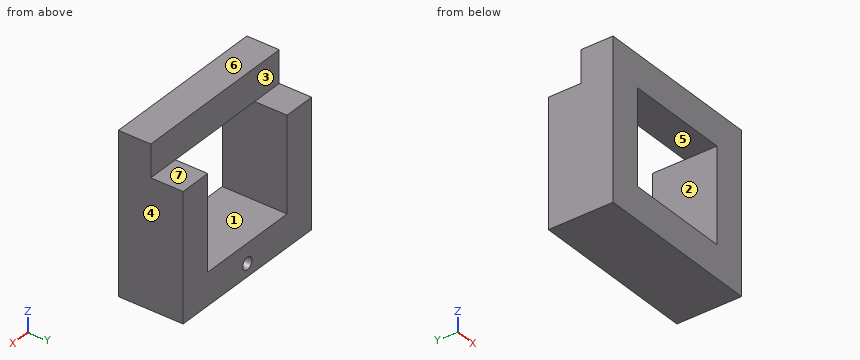
Autodesk Inventor part; units mm, degrees
ref_plane "YZ Plane" through (0, 0, 0) normal (1, 0, 0) x (0, 1, 0)
ref_plane "XZ Plane" through (0, 0, 0) normal (0, 1, 0) x (-1, 0, 0)
ref_plane "XY Plane" through (0, 0, 0) normal (0, 0, 1) x (1, 0, 0)
sketch "Sketch1" plane through (0, 0, 0) normal (0, 1, 0) x (-1, 0, 0)
  line L0 (8.1915, 7.4295) -> (-8.1915, 7.4295)
  line L1 (-8.1915, 7.4295) -> (-8.1915, -7.4295)
  line L2 (-8.1915, -7.4295) -> (8.1915, -7.4295)
  line L3 (8.1915, -7.4295) -> (8.1915, 7.4295)
  line L4 (13.2715, -12.5095) -> (-13.2715, -12.5095)
  line L5 (-13.2715, -12.5095) -> (-13.2715, 12.5095)
  line L6 (-13.2715, 12.5095) -> (13.2715, 12.5095)
  line L7 (13.2715, 12.5095) -> (13.2715, -12.5095)
  point P0 (0, 0)
  point P1 (0, -7.4295)
  point P2 (8.1915, 0)
  dimension "d0" = 16.383
  dimension "d1" = 14.859
  dimension "d2" = 5.08
extrude "Extrusion1" add sketch "Sketch1" along normal blind 5.08
sketch "Sketch2" plane through (0, 5.08, 0) normal (0, 1, 0) x (1, 0, 0)
  line L0 (-13.2715, -12.5095) -> (13.2715, -12.5095)
  line L1 (13.2715, -12.5095) -> (13.2715, 12.5095)
  line L2 (13.2715, 12.5095) -> (-13.2715, 12.5095)
  line L3 (-13.2715, 12.5095) -> (-13.2715, -12.5095)
  line L4 (-8.1915, -7.4295) -> (-8.1915, 7.4295)
  line L5 (-8.1915, 7.4295) -> (8.1915, 7.4295)
  line L6 (8.1915, 7.4295) -> (8.1915, -7.4295)
  line L7 (8.1915, -7.4295) -> (-8.1915, -7.4295)
  line L8 (-8.1915, -7.4295) -> (-13.2715, -7.4295)
  line L9 (8.1915, -7.4295) -> (-8.1915, -7.4295)
  line L10 (8.1915, -7.4295) -> (13.2715, -7.4295)
  point P0 (0, 0)
extrude "Extrusion2" add sketch "Sketch2" along normal blind 5.08 contours L3 L2 L1 L10 L6 L5 L4 L8
sketch "Sketch3" plane through (0, 10.16, 0) normal (0, 1, 0) x (1, 0, 0)
  line L0 (-8.1915, 7.4295) -> (8.1915, 7.4295)
  line L1 (-3.81, 7.4295) -> (3.81, 7.4295) construction
  line L2 (3.81, 7.4295) -> (3.81, 9.7155) construction
  line L3 (3.81, 9.7155) -> (-3.81, 9.7155) construction
  line L4 (-3.81, 9.7155) -> (-3.81, 7.4295) construction
  circle A0 centre (0, 10.4775) radius 1.143 construction
  circle A1 centre (0, 10.4775) radius 0.9525
  point P0 (0, 0)
  point P1 (0, 9.7155)
  point P2 (0, 7.4295)
  point P3 (0, 7.4295)
  dimension "d7" = 7.62
  dimension "d8" = 2.286
  dimension "d9" = 2.286
  dimension "d10" = 1.905
  dimension "d14" = 0.762
extrude "Extrusion3" cut sketch "Sketch3" against normal blind 6.35
properties part number "RJ45Adapter"
Geometry check sheet. Reference: the model listing, model coordinates, mm. Face numbers are marked on the shaded views. A direction names the side the tool comes from. Give positions to 0.01 mm unless a question says otherwise; leave off trailing zeros. Write each loop counter-clockwise with the first axis right and the second up, starting at its lowest first coordinate (ties: lowest second). Pieces come first, ordered by that corner, then holes. Notation, with made-up numbers: (29.25, -20) -> (71.25, -20) arc R22 ccw to (71.25, -6) -> close; hole circle Ø11 at (52.25, 72). An arc over 180 degrees is marked (long way). One line per question, with ' | ' between items.
Item 1: Sectioned sample at D-D, the plane x = -11.25. Record the boundary of the cut face in (y, z).
Determined:
outline: (0, -12.51) -> (10.16, -12.51) -> (10.16, 7.43) -> (5.08, 7.43) -> (5.08, 12.51) -> (0, 12.51) -> close
Item 2: Draft check along X on the marked faces 1, 2, 3 and 4. Enter one of: released by +X, released by -X, zero draft, split by the parting line, or undercut.
Determined:
face 1: undercut | face 2: undercut | face 3: zero draft | face 4: released by +X
Item 3: Sectioned sample at B-B, the plane x = 6.5. Record the boundary of the cut face in (y, z), plus the area to 3 significant figures.
Determined:
outline: (0, -12.51) -> (10.16, -12.51) -> (10.16, -7.43) -> (0, -7.43) -> close; (0, 7.43) -> (5.08, 7.43) -> (5.08, 12.51) -> (0, 12.51) -> close | area: 77.4 mm^2
Item 4: Sectioned sample at C-C, the plane y = 1.25. Record the boundary of the cut face in (x, z), plus the area to 3 significant figures.
Determined:
outline: (-13.27, -12.51) -> (13.27, -12.51) -> (13.27, 12.51) -> (-13.27, 12.51) -> close; hole (-8.19, -7.43) -> (8.19, -7.43) -> (8.19, 7.43) -> (-8.19, 7.43) -> close | area: 421 mm^2
Item 5: Depth check by flat-ended pin: pin 1 (4 mm diameter, centred on x = -5, z = 7, fed in from +Y); pin 2 (2 mm diameter, centred on x = -4.5, y = 7.5, fed in from +Z); pin 3 (2.5 mm diameter, centred on x = -11.5, y = 8.5, fed in from +Z). Enter the tip coordinate at first touch or a pass-through.
Determined:
pin 1: y = 5.08 | pin 2: z = -7.43 | pin 3: z = 7.43
Item 6: Access from +Z, -Z, +X, -X, +Y, -Y to the whole of each face (thin tool, end or side, straight path). Record for the marked faces 5, 6 and 7.
Determined:
face 5: +Y, -Y | face 6: +Z, +X, -X, +Y, -Y | face 7: +Z, +X, -X, +Y
Item 7: Sectioned sample at A-A, the plane z = -4.5. Record the boundary of the cut face in (x, y), plus the area to 3 significant figures.
Determined:
outline: (-13.27, 0) -> (-8.19, 0) -> (-8.19, 10.16) -> (-13.27, 10.16) -> close; (8.19, 0) -> (13.27, 0) -> (13.27, 10.16) -> (8.19, 10.16) -> close | area: 103 mm^2
Item 8: Scan lines: line 1 along X through (y, z) = (4.25, 5); line 2 along Z through (x, y) = (0, 5.75) (1 decimal); line 3 along Z through (x, y) = (-7.25, 6.75). Record each from-to range of solid material in increasing order.
Determined:
line 1: -13.27 to -8.19, 8.19 to 13.27 | line 2: -12.5 to -11.4, -9.5 to -7.4 | line 3: -12.51 to -7.43
